from build123d import *

# Parameters (mm, degrees)
BOSS_EXTRUDE1_DEPTH = 156.2
SKETCH5_R           = 10
CUT_EXTRUDE1_DEPTH  = 101
SKETCH6_R           = 25
CUT_EXTRUDE2_DEPTH  = 101.0000001


with BuildPart() as part:
    # Sketch1 → Boss-Extrude1 (new body)
    with BuildSketch(Plane(origin=(0, 0, 0), x_dir=(1, 0, 0), z_dir=(0, 1, 0))):
        with BuildLine():
            ThreePointArc((139.891219134, -157.482137257), (-0.054560073, -162.999999162), (-140, -157.473539028))
            Line((-140, -157.473539028), (-140, -257.473539028))
            Line((-140, -257.473539028), (-74.996125665, -257.473539028))
            ThreePointArc((-74.996125665, -257.473539028), (0, -183.235861256), (74.996125665, -257.473539028))
            Line((74.996125665, -257.473539028), (139.891219134, -257.473539028))
            Line((139.891219134, -257.473539028), (139.891219134, -157.482137257))
        make_face()
    extrude(amount=BOSS_EXTRUDE1_DEPTH)

    # Sketch5 → Cut-Extrude1 (cut, through all)
    with BuildSketch(Plane.XY.offset(257.473539028)):
        with Locations((107.4436724, 136.2)):
            Circle(SKETCH5_R)
        with Locations((107.4436724, 20)):
            Circle(SKETCH5_R)
        with Locations((-107.4436724, 20)):
            Circle(SKETCH5_R)
        with Locations((-107.4436724, 136.2)):
            Circle(SKETCH5_R)
    extrude(amount=-CUT_EXTRUDE1_DEPTH, mode=Mode.SUBTRACT)

    # Sketch6 → Cut-Extrude2 (cut, through all)
    with BuildSketch(Plane.XY.offset(257.473539028)):
        with Locations((0, 78.1)):
            Circle(SKETCH6_R)
    extrude(amount=-CUT_EXTRUDE2_DEPTH, mode=Mode.SUBTRACT)


solid = part.part
Verification items for the finished model (mm, model axes). Coordinates: 2 decimals unless noted, no trailing zeros. Order: outer loops, then holes, each group sorted by start corner. A loop starts at its lowest first (then second) coordinate and runs counter-clockwise, first axis right, second up. Notation, with made-up numbers: M 47.5,16 L 65.5,16 A15 cw 65.5,42 Z; hole C -5,44.5 d1. An arc over 180 degrees is marked long. One line per item, written item: value. Start each with the question number.
Item 1: Depth check by flat-ended pin: P1, Ø23, axis at x = -107.44, y = 20, coming from the +Z side; P2, Ø16, axis at x = -107.44, y = 136.2, coming from the -Z side; P3, Ø6, axis at x = -84.5, y = 100.5, coming from the -Z side. Enter the tip coordinate at first touch or a pass-through.
Item 2: Sectioned sample at C-C on z = 241. Record the cut outline in (x, y), then the cut area to 3 significant figures.
Item 3: Thickness scan on probe 1 along Y at (x, z) = (114.5, 211.5); probe 2 along X at (y, z) = (136.2, 222); probe 3 along X at (y, z) = (136.2, 223.5). Record the ranges inside material, lowest first.
Item 4: Mould release check, pull along Y, two halves, no side actions. Record for faces 1 (the cylindrical face through (105.276, 126.438, 208.982)), 2 (the flat face through (-2, 0, 173)), 3 (the flat face through (139.891, 77, 208)), 4 (the cylindrical face through (100.073, 26.758, 208.982)): pulls with the +Y half, pulls with the -Y half, needs draft (parallel to the pull), parting line crosses it, or undercut.
Item 5: Sectioned sample at B-B on y = 78.1. Record the cut outline in (x, z).
Item 6: Sectioned sample at A-A on x = 0. Record the cut outline in (y, z), then the cut area to 3 significant figures.
Item 7: Sectioned sample at D-D on z = 177.5. Record the cut outline in (x, y).
Calculated:
1. P1: z = 257.47
1. P2: through
1. P3: z = 160.84
2. outline: M -140,0 L -72.99,0 L -72.99,156.2 L -140,156.2 Z; M 72.99,0 L 139.89,0 L 139.89,156.2 L 72.99,156.2 Z; hole C -107.44,20 d20; hole C -107.44,136.2 d20; hole C 107.44,20 d20; hole C 107.44,136.2 d20
2. area: 19,700 mm^2
3. probe 1: 0 to 12.91, 27.09 to 129.11, 143.29 to 156.2
3. probe 2: -140 to -117.44, -97.44 to -65.67, 65.67 to 97.44, 117.44 to 139.89
3. probe 3: -140 to -117.44, -97.44 to -66.47, 66.47 to 97.44, 117.44 to 139.89
4. face 1: undercut
4. face 2: pulls with the -Y half
4. face 3: needs draft
4. face 4: undercut
5. outline: M -140,157.47 A1776.05 cw -25,162.82 L -25,187.53 A75 cw -75,257.47 L -140,257.47 Z; M 25,162.82 A1776.05 cw 139.89,157.48 L 139.89,257.47 L 75,257.47 A75 cw 25,187.53 Z
6. outline: M 0,163 L 53.1,163 L 53.1,183.24 L 0,183.24 Z; M 103.1,163 L 156.2,163 L 156.2,183.24 L 103.1,183.24 Z
6. area: 2,150 mm^2
7. outline: M -140,0 L 139.89,0 L 139.89,156.2 L -140,156.2 Z; hole C -107.44,20 d20; hole C -107.44,136.2 d20; hole C 0,78.1 d50; hole C 107.44,20 d20; hole C 107.44,136.2 d20
